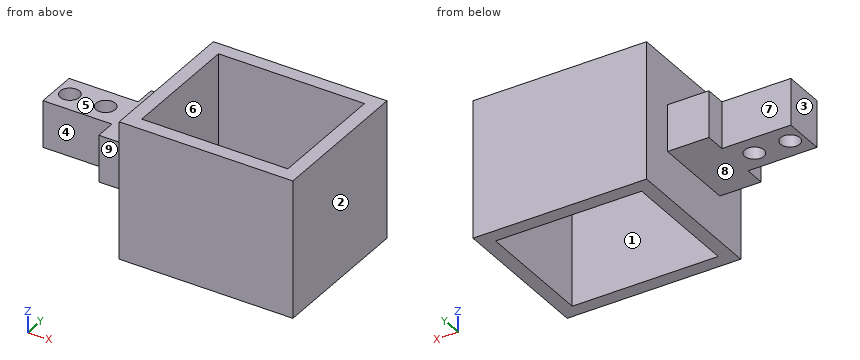
Autodesk Inventor part; units mm, degrees
ref_plane "YZ Plane" through (0, 0, 0) normal (1, 0, 0) x (0, 1, 0)
ref_plane "XZ Plane" through (0, 0, 0) normal (0, 1, 0) x (-1, 0, 0)
ref_plane "XY Plane" through (0, 0, 0) normal (0, 0, 1) x (1, 0, 0)
sketch "Sketch1" plane through (0, 0, 0) normal (1, 0, 0) x (0, 1, 0)
  line L0 (-15, 8.5) -> (15, 8.5)
  line L1 (15, 8.5) -> (15, -8.5)
  line L2 (15, -8.5) -> (-15, -8.5)
  line L3 (-15, -8.5) -> (-15, 8.5)
  line L4 (-15, 8.5) -> (15, -8.5) construction
  line L5 (15, 8.5) -> (-15, -8.5) construction
  point P0 (0, 0)
  dimension "d0" = 30
  dimension "d1" = 17
extrude "Extrusion1" add sketch "Sketch1" along normal blind 15
sketch "Sketch2" plane through (0, 0, 0) normal (-1, 0, 0) x (0, 0, 1)
  line L0 (-8.5, 7.5) -> (8.5, 7.5)
  line L1 (8.5, 7.5) -> (8.5, -7.5)
  line L2 (8.5, -7.5) -> (-8.5, -7.5)
  line L3 (-8.5, -7.5) -> (-8.5, 7.5)
  line L4 (-8.5, 7.5) -> (8.5, -7.5) construction
  line L5 (8.5, 7.5) -> (-8.5, -7.5) construction
  point P0 (0, 0)
  dimension "d4" = 17
  dimension "d5" = 15
extrude "Extrusion2" add sketch "Sketch2" along normal blind 25
sketch "Sketch3" plane through (15, 0, 0) normal (1, 0, 0) x (0, 0, -1)
  line L0 (-25, 27) -> (25, 27)
  line L1 (25, 27) -> (25, -27)
  line L2 (25, -27) -> (-25, -27)
  line L3 (-25, -27) -> (-25, 27)
  line L4 (-25, 27) -> (25, -27) construction
  line L5 (25, 27) -> (-25, -27) construction
  point P0 (0, 0)
  dimension "d8" = 50
  dimension "d9" = 54
extrude "Extrusion3" add sketch "Sketch3" along normal blind 5
sketch "Sketch4" plane through (20, 0, 0) normal (1, 0, 0) x (0, 0, -1)
  line L0 (-25, 27) -> (-25, -27)
  line L1 (-25, 27) -> (25, 27)
  line L2 (25, 27) -> (25, 22)
  line L3 (25, 22) -> (-25, 22)
  line L4 (-25, 22) -> (-25, 27)
  line L5 (-25, -27) -> (25, -27)
  line L6 (-25, -27) -> (25, -27)
  line L7 (25, -27) -> (25, -22)
  line L8 (25, -22) -> (-25, -22)
  line L9 (-25, -22) -> (-25, -27)
  point P0 (0, 0)
  dimension "d12" = 50
  dimension "d13" = 5
  dimension "d14" = 50
  dimension "d15" = 5
extrude "Extrusion4" add sketch "Sketch4" along normal blind 58
sketch "Sketch5" plane through (20, -22, 25) normal (0, 1, 0) x (1, 0, 0)
  line L0 (0, 50) -> (58, 50)
  line L1 (0, 0) -> (58, 0)
  line L2 (58, 50) -> (53, 50)
  line L3 (53, 50) -> (53, 0)
  line L4 (53, 0) -> (58, 0)
  line L5 (58, 0) -> (58, 50)
  point P0 (-20, 25)
  dimension "d18" = 5
extrude "Extrusion5" add sketch "Sketch5" along normal blind 45
sketch "Sketch6" plane through (15, -27, 25) normal (0, 0, 1) x (1, 0, 0)
  point P0 (-15, 27)
sketch "Sketch7" plane through (0, 7.5, 8.5) normal (0, 0, 1) x (1, 0, 0)
  line L0 (-25, 0) -> (-25, -15)
  line L1 (-25, -7.5) -> (-20, -7.5)
  line L2 (0, -7.5) -> (-7, -7.5)
  circle A0 centre (-7, -7.5) radius 3.5
  circle A1 centre (-20, -7.5) radius 3.5
  dimension "d21" = 5
  dimension "d22" = 7
  dimension "d23" = 7
  dimension "d24" = 7
extrude "Extrusion6" cut sketch "Sketch7" against normal through all
sketch "Sketch8" plane through (0, -15, -8.5) normal (0, 0, -1) x (-1, 0, 0)
  point P0 (0, 15)
properties part number "Upper_battery"
Here's how the part is built. I have some questions about the finished solid (model axes, mm). Face numbers are marked on the shaded views. A direction names the side the tool comes from. Give positions to 0.01 mm unless a question says otherwise; leave off trailing zeros. Order: outer loops, then holes, each group sorted by start corner. A loop starts at its lowest first (then second) coordinate and runs counter-clockwise, first axis right, second up. Notation, with made-up numbers: (23, 18.25) - (66, 18.25) arc R31 cw to (66, 56.25) - close; hole circle Ø3 at (73, 22). An arc over 180 degrees is marked (long way). Answer as a JSON object with one key per item and string values. Group by question number.
Item 1: If we mould it in two halves opening along X, with no side actions, what happens to the marked faces 1, 2, 3 and 4? For each: pulls with the +X half, pulls with the -X half, needs draft (parallel to the pull), parting line crosses it, or undercut.
Item 2: If we section it at C-C on x = 34.5: Please give me the cut outline in (y, z).
Item 3: If we section it at D-D on y = 0: Please give me the cut outline in (x, z), and give its area (3 significant figures).
Item 4: Which directions (+Z, -Z, +X, -X, +Y, -Y) give clear straight access to the entire face, cutting with the end or side of a thin tool? Please do the marked faces 5, 6, 7, 8 and 9.
Item 5: Please list where these lines run through material, in increasing order: probe 1 along Y at (x, z) = (56.5, 5.5); probe 2 along X at (y, z) = (20.5, 3.5); probe 3 along X at (y, z) = (-5, -3).
Item 6: If we section it at A-A on y = 11: Please give me the cut outline in (x, z), and give its area (3 significant figures).
Item 7: For P1, Ø4, axis at y = -3.5, z = -15, coming from the -X side; P2, Ø6.5, axis at x = -7, y = 0, coming from the -Z side; P3, Ø15, axis at x = -4, y = 4.5, coming from the -Z side; P4, Ø9, axis at x = -15, y = 1.5, coming from the +Z side, each with a flat end and sliding along its axis, tell me the tip position at first contact or that it passes through.
Item 8: If we section it at B-B on z = -0.5: Please give me the cut outline in (x, y).
Result set:
{
 "1": {"face 1": "undercut", "face 2": "pulls with the +X half", "face 3": "pulls with the -X half", "face 4": "needs draft"},
 "2": {"outline": "(-27, -25) - (-22, -25) - (-22, 25) - (-27, 25) - close; (22, -25) - (27, -25) - (27, 25) - (22, 25) - close"},
 "3": {"outline": "(-25, -8.5) - (-23.5, -8.5) - (-23.5, 8.5) - (-25, 8.5) - close; (-16.5, -8.5) - (-10.5, -8.5) - (-10.5, 8.5) - (-16.5, 8.5) - close; (-3.5, -8.5) - (15, -8.5) - (15, -25) - (20, -25) - (20, 25) - (15, 25) - (15, 8.5) - (-3.5, 8.5) - close; (73, -25) - (78, -25) - (78, 25) - (73, 25) - close", "area": "942 mm²"},
 "4": {"face 5": "+Z, -X, +Y, -Y", "face 6": "+Z, -Z", "face 7": "+Z, -Z, -X, +Y", "face 8": "-Z, -X, +Y, -Y", "face 9": "+Z, -Z, -X, -Y"},
 "5": {"probe 1": "-27 to -22, 22 to 27", "probe 2": "15 to 20, 73 to 78", "probe 3": "-25 to 20, 73 to 78"},
 "6": {"outline": "(0, -8.5) - (15, -8.5) - (15, -25) - (20, -25) - (20, 25) - (15, 25) - (15, 8.5) - (0, 8.5) - close; (73, -25) - (78, -25) - (78, 25) - (73, 25) - close", "area": "755 mm²"},
 "7": {"P1": "x = 15", "P2": "through", "P3": "z = -8.5", "P4": "z = 8.5"},
 "8": {"outline": "(-25, -7.5) - (0, -7.5) - (0, -15) - (15, -15) - (15, -27) - (78, -27) - (78, 27) - (15, 27) - (15, 15) - (0, 15) - (0, 7.5) - (-25, 7.5) - close; hole circle Ø7 at (-20, 0); hole circle Ø7 at (-7, 0); hole (20, -22) - (73, -22) - (73, 22) - (20, 22) - close"}
}
